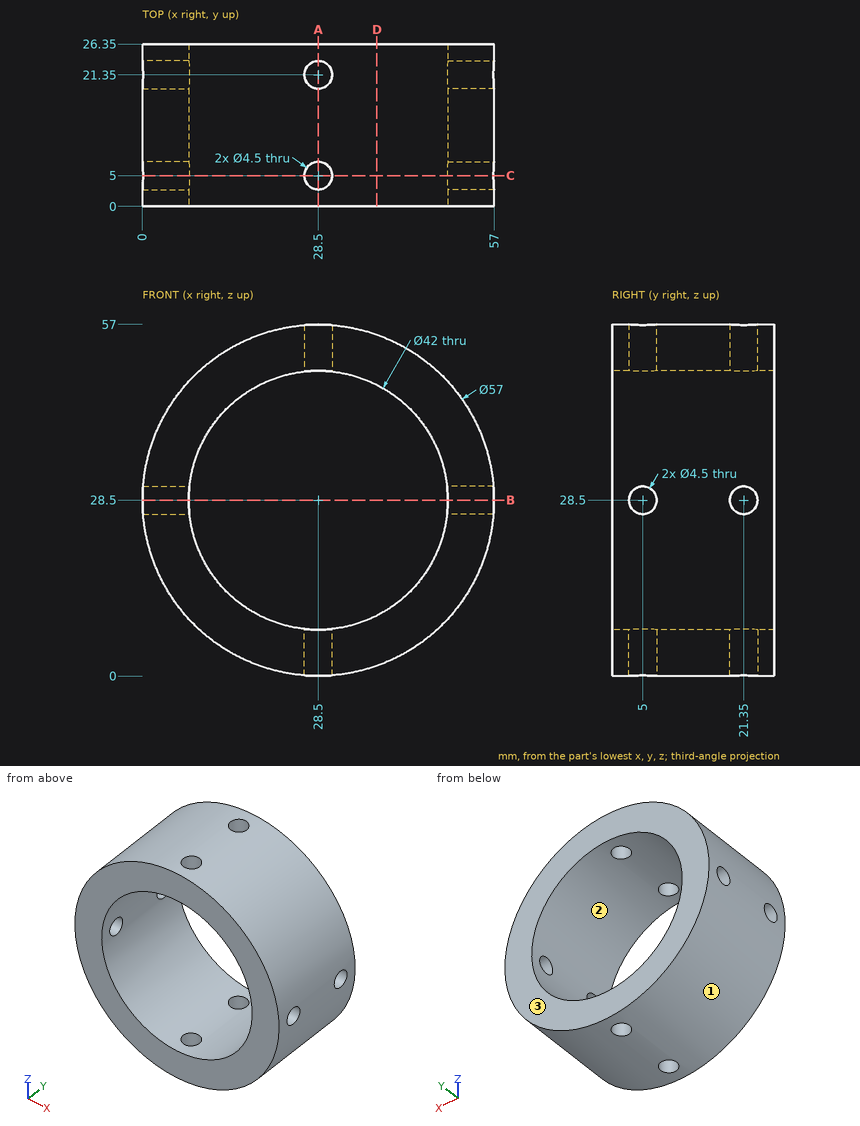
Part print with two shaded views. Sizes in mm from the minimum x, y, z corner. Round coordinates to 2 decimals unless told otherwise and drop trailing zeros. Order: outer loops, then holes, each group sorted by start corner. A loop starts at its lowest first (then second) coordinate and runs counter-clockwise, first axis right, second up. Notation, with made-up numbers: M -3.5,52.25 L 37.5,52.25 A19 ccw 37.5,86.25 Z; hole C 59,81 d1. An arc over 180 degrees is marked long. Put each result on its own line as item: value. Start each with the question number.
1. Drill centre lines: probe 1 along Y at (x, z) = (28, 54); probe 2 along Z at (x, y) = (16, 18.75); probe 3 along Z at (x, y) = (18.5, 25.25). Where is each one in solid material? Low to high. Write a range as [from, to].
2. Two-plate mould, pull along X, no slides. Class the marked faces 1, 2 and 3: +X half, -X half, draft (parallel to the pull), parting line (faces both ways), or undercut.
3. Slice it at C-C on y = 5. List the corners of the cut face in (x, z).
4. Drop flat-ended pins along their axis: pin 1 (8 mm diameter, centred on y = 23.5, z = 23.5, fed in from +X); pin 2 (2 mm diameter, centred on y = 22.5, z = 16.5, fed in from -X); pin 3 (3 mm diameter, centred on y = 23, z = 38.5, fed in from -X). Give the stop position or say it passes through.
5. Slice it at D-D on x = 38. List the corners of the cut face in (y, z), then the cut area to 3 significant figures.
6. Slice it at B-B on z = 28.5. List the corners of the cut face in (x, y).
7. Slice it at A-A on x = 28.5. List the corners of the cut face in (y, z), then the cut area to 3 significant figures.
Findings:
1. probe 1: [0, 2.81], [7.19, 19.16], [23.54, 26.35]
1. probe 2: [2.89, 11.63], [45.37, 54.11]
1. probe 3: [1.81, 10.03], [46.97, 55.19]
2. face 1: parting line
2. face 2: undercut
2. face 3: draft
3. outline: M 0.09,26.25 A28.5 ccw 26.25,0.09 L 26.25,7.62 A21 cw 7.62,26.25 Z; M 0.09,30.75 L 7.62,30.75 A21 cw 26.25,49.38 L 26.25,56.91 A28.5 ccw Z; M 30.75,0.09 A28.5 ccw 56.91,26.25 L 49.38,26.25 A21 cw 30.75,7.62 Z; M 30.75,49.38 A21 cw 49.38,30.75 L 56.91,30.75 A28.5 ccw 30.75,56.91 Z
4. pin 1: x = 56.98
4. pin 2: x = 2.21
4. pin 3: x = 1.3
5. outline: M 0,1.63 L 26.35,1.63 L 26.35,9.77 L 0,9.77 Z; M 0,47.23 L 26.35,47.23 L 26.35,55.37 L 0,55.37 Z
5. area: 429 mm2
6. outline: M 0,0 L 7.5,0 L 7.5,2.75 L 0,2.75 Z; M 0,7.25 L 7.5,7.25 L 7.5,19.1 L 0,19.1 Z; M 0,23.6 L 7.5,23.6 L 7.5,26.35 L 0,26.35 Z; M 49.5,0 L 57,0 L 57,2.75 L 49.5,2.75 Z; M 49.5,7.25 L 57,7.25 L 57,19.1 L 49.5,19.1 Z; M 49.5,23.6 L 57,23.6 L 57,26.35 L 49.5,26.35 Z
7. outline: M 0,0 L 2.75,0 L 2.75,7.5 L 0,7.5 Z; M 0,49.5 L 2.75,49.5 L 2.75,57 L 0,57 Z; M 7.25,0 L 19.1,0 L 19.1,7.5 L 7.25,7.5 Z; M 7.25,49.5 L 19.1,49.5 L 19.1,57 L 7.25,57 Z; M 23.6,0 L 26.35,0 L 26.35,7.5 L 23.6,7.5 Z; M 23.6,49.5 L 26.35,49.5 L 26.35,57 L 23.6,57 Z
7. area: 260 mm2
